Job drawing, mm, ordinate dimensions from the low corner. One solid piece. A direction names the side the tool comes from. Coordinates: 2 decimals unless noted, no trailing zeros. Write each loop counter-clockwise with the first axis right and the second up, starting at its lowest first coordinate (ties: lowest second). Pieces come first, ordered by that corner, then holes. Notation, with made-up numbers: (43, 76.25) -> (64, 76.25) arc R19 cw to (64, 95.25) -> close; hole circle Ø4 at (63, -35.5). An arc over 180 degrees is marked (long way). One line per question, with ' | ' between items. Start each with the question number.
Item 1: Saw through at B-B (z = 25). List the corners of the cut face in (x, y).
Item 2: Saw through at C-C (y = 5.5). List the corners of the cut face in (x, z), and give its area (3 significant figures).
Item 3: Pin check, flat tips, straight feed: pin 1 (20 mm diameter, centred on y = 30.5, z = 25, fed in from -X); pin 2 (14.5 mm diameter, centred on y = 37, z = 37, fed in from +X); pin 3 (1 mm diameter, centred on x = 42.5, z = 24, fed in from +Y). Stop position of each tip, or through.
Item 4: Probe probe 1 along Y at (x, z) = (2.3, 25); probe 2 along Z at (x, y) = (2, 30); probe 3 along Y at (x, z) = (19, 17). List the from-to ranges inside material, lowest first. Write a range as [from, to].
Item 5: 3-axis set-ups, long thin cutter, end or side, ignore diameter. For the marked faces 1 and 2: which of +Z, -Z, +X, -X, +Y, -Y reach the whole face in a straight line?
Item 6: Saw through at A-A (y = 30.5). List the corners of the cut face in (x, z), and give its area (3 significant figures).
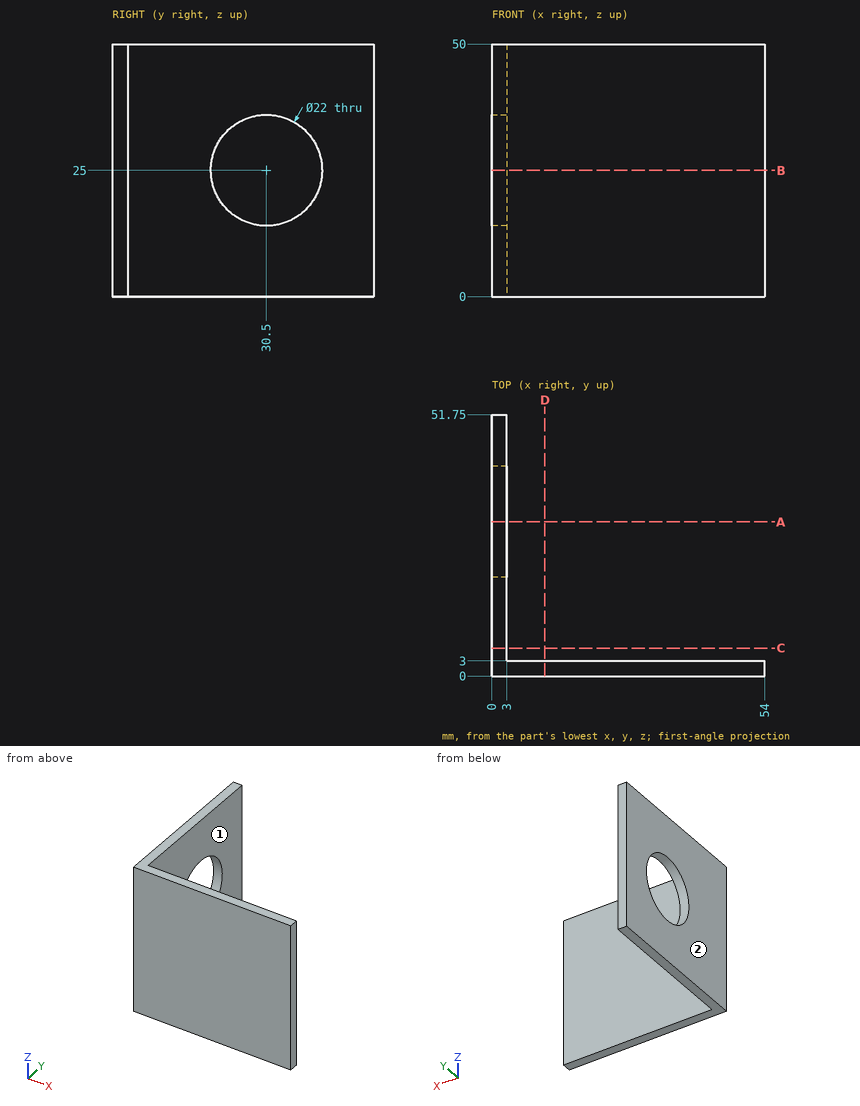
From the geometry:
1) outline: (0, 0) -> (54, 0) -> (54, 3) -> (3, 3) -> (3, 19.5) -> (0, 19.5) -> close; (0, 41.5) -> (3, 41.5) -> (3, 51.75) -> (0, 51.75) -> close
2) outline: (0, 0) -> (3, 0) -> (3, 50) -> (0, 50) -> close | area: 150 mm2
3) pin 1: through | pin 2: x = 3 | pin 3: y = 3
4) probe 1: [0, 19.5], [41.5, 51.75] | probe 2: [0, 14.01], [35.99, 50] | probe 3: [0, 3]
5) face 1: +Z, -Z, +X, +Y | face 2: +Z, -Z, -X, +Y, -Y
6) outline: (0, 0) -> (3, 0) -> (3, 14) -> (0, 14) -> close; (0, 36) -> (3, 36) -> (3, 50) -> (0, 50) -> close | area: 84.0 mm2
